Job drawing, mm, ordinate dimensions from the low corner. One solid piece. A direction names the side the tool comes from. Round coordinates to 2 decimals unless told otherwise and drop trailing zeros. Write each loop counter-clockwise with the first axis right and the second up, starting at its lowest first coordinate (ties: lowest second). Pieces come first, ordered by that corner, then holes. Notation, with made-up numbers: M 76,39 L 116,39 A28 ccw 116,76 Z; hole C -22,-6.5 d8. An arc over 180 degrees is marked long. Answer as a JSON object with one key per item and string values. Group by question number.
1. Band-saw the part on B-B, the plane z = 13.5. Write the cut outline in (x, y).
2. Drill centre lines: line 1 (X direction, y = 17.5, z = 10); line 2 (X direction, y = 1.5, z = 14.3); line 3 (Y direction, x = 2.25, z = 10.5). Where is each one in solid material? Low to high. Write a range as from..to.
3. Which spindle directions (+Z, -Z, +X, -X, +Y, -Y) get a long thin tool onto all of the face, cutting with end or side? Do the marked faces 1 and 2. Say none if no direction does.
4. Band-saw the part on A-A, the plane x = 9.5. Write the cut outline in (y, z), plus the area to 3 significant figures.
5. Drop flat-ended pins along their axis: pin 1 (2 mm diameter, centred on y = 9, z = 14, fed in from +X); pin 2 (1 mm diameter, centred on x = 16, z = 17, fed in from +Y); pin 3 (3 mm diameter, centred on x = 2.5, y = 2.5, fed in from +Z); pin 4 (1.5 mm diameter, centred on x = 3.03, z = 14.3, fed in from +Y). Give the stop position or say it passes through.
6. Band-saw the part on C-C, the plane x = 13.25. Write the cut outline in (y, z), plus the area to 3 significant figures.
7. Band-saw the part on D-D, the plane z = 11. Write the cut outline in (x, y).
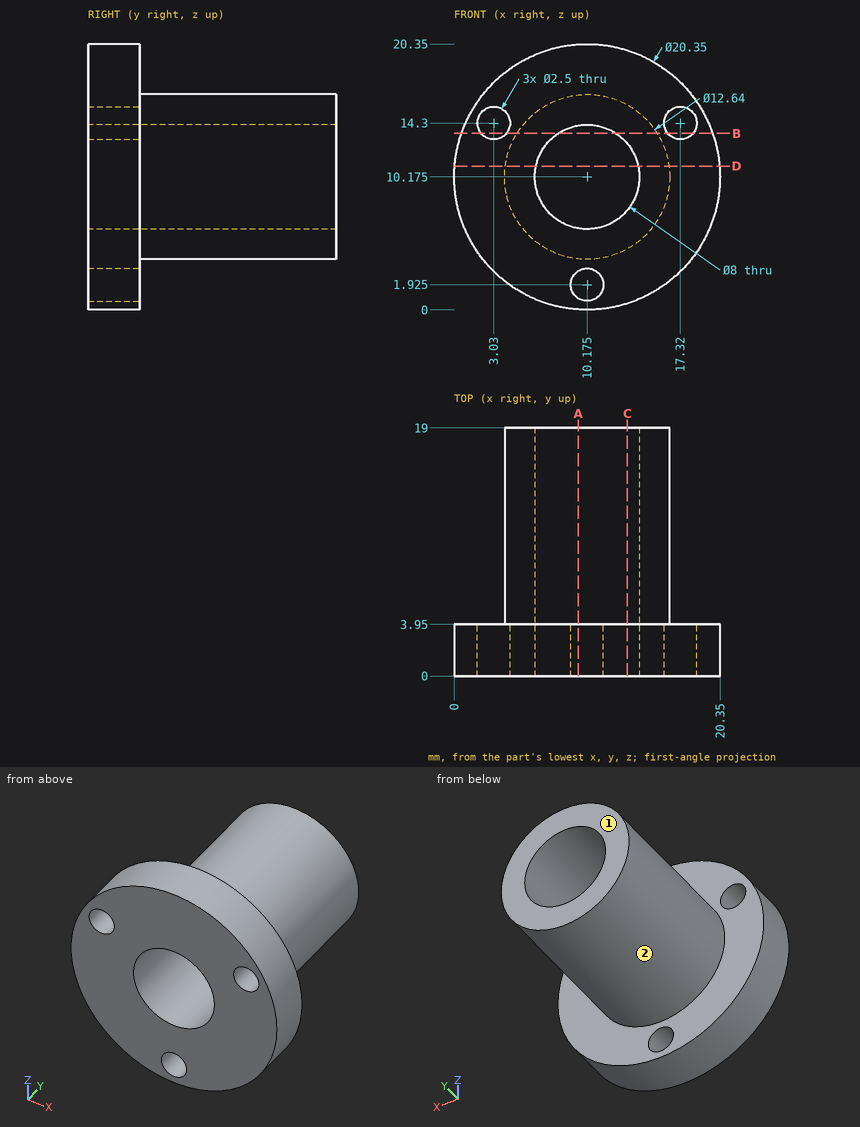
Worked answers:
{
 "1": {"outline": "M 0.56,0 L 2.07,0 L 2.07,3.95 L 0.56,3.95 Z; M 3.99,0 L 7.95,0 L 7.95,19 L 4.8,19 L 4.8,3.95 L 3.99,3.95 Z; M 12.4,0 L 16.36,0 L 16.36,3.95 L 15.55,3.95 L 15.55,19 L 12.4,19 Z; M 18.28,0 L 19.79,0 L 19.79,3.95 L 18.28,3.95 Z"},
 "2": {"line 1": "x = 3.86..6.18, 14.17..16.49", "line 2": "x = 0.87..1.78, 4.28..16.07, 18.57..19.48", "line 3": "y = 0..3.95"},
 "3": {"face 1": "+Z, -Z, +X, -X, +Y", "face 2": "+Y"},
 "4": {"outline": "M 0,0.02 L 3.95,0.02 L 3.95,0.87 L 0,0.87 Z; M 0,2.98 L 3.95,2.98 L 3.95,3.89 L 19,3.89 L 19,6.23 L 0,6.23 Z; M 0,14.12 L 19,14.12 L 19,16.46 L 3.95,16.46 L 3.95,20.33 L 0,20.33 Z", "area": "111 mm^2"},
 "5": {"pin 1": "stops at x = 15.83", "pin 2": "stops at y = 3.95", "pin 3": "stops at z = 18.26", "pin 4": "passes through"},
 "6": {"outline": "M 0,0.48 L 3.95,0.48 L 3.95,4.65 L 19,4.65 L 19,7.62 L 0,7.62 Z; M 0,12.73 L 19,12.73 L 19,15.7 L 3.95,15.7 L 3.95,19.87 L 0,19.87 Z", "area": "146 mm^2"},
 "7": {"outline": "M 0.03,0 L 6.26,0 L 6.26,19 L 3.91,19 L 3.91,3.95 L 0.03,3.95 Z; M 14.09,0 L 20.32,0 L 20.32,3.95 L 16.44,3.95 L 16.44,19 L 14.09,19 Z"}
}
